Drawing for the job (mm, zero at the part's lowest x, y, z). A direction names the side the tool comes from. Coordinates: 2 decimals unless noted, no trailing zeros. Write each loop counter-clockwise with the first axis right and the second up, starting at its lowest first coordinate (ties: lowest second). Pieces come first, ordered by that corner, then holes. Notation, with made-up numbers: (11.25, -4.5) - (35.25, -4.5) arc R31 cw to (35.25, 31.5) - close; hole circle Ø2 at (42, -4). An arc over 180 degrees is marked (long way). Write each question's results on one line, items separated by ' | '.
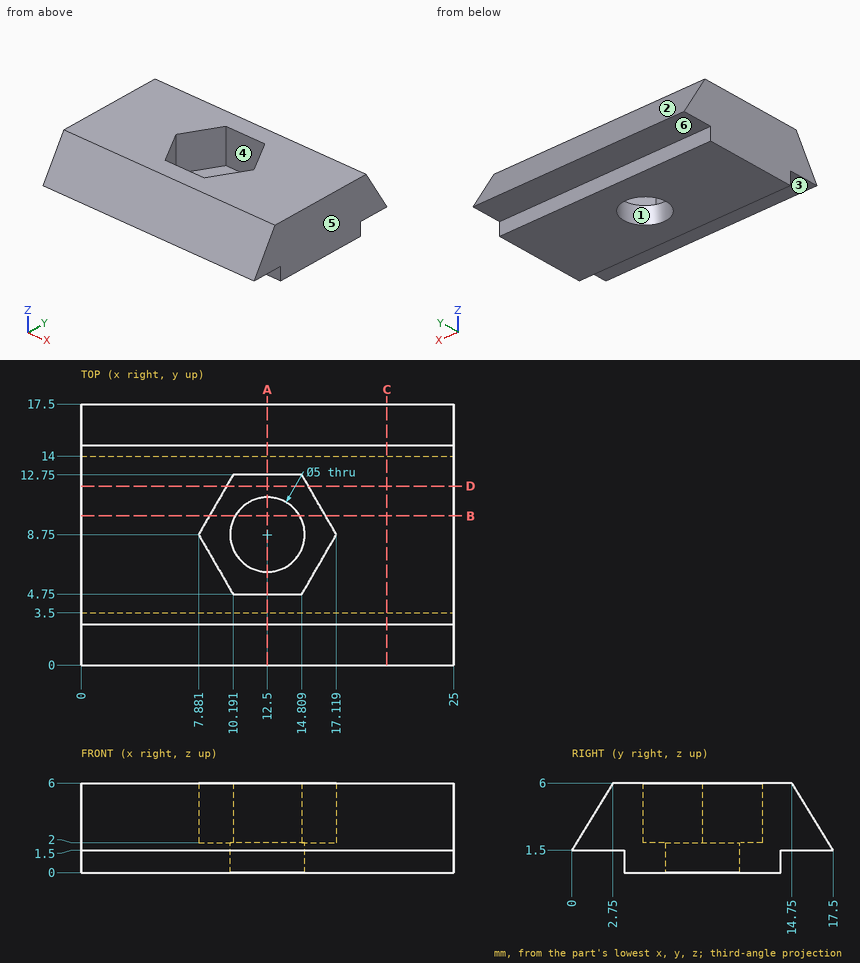
(1) Wall check: line 1 (X direction, y = 8.75, z = 0.8); line 2 (Z direction, x = 21.25, y = 14.5); line 3 (Y direction, x = 16, z = 0.75). Give the ranges that are in metal, low to high. Write a range as from..to.
Return value:
line 1: x = 0..10, 15..25 | line 2: z = 1.5..6 | line 3: y = 3.5..14
(2) Saw through at A-A on x = 12.5. Write the cut outline in (y, z).
Return value:
outline: (0, 1.5) - (3.5, 1.5) - (3.5, 0) - (6.25, 0) - (6.25, 2) - (4.75, 2) - (4.75, 6) - (2.75, 6) - close; (11.25, 0) - (14, 0) - (14, 1.5) - (17.5, 1.5) - (14.75, 6) - (12.75, 6) - (12.75, 2) - (11.25, 2) - close
(3) Saw through at C-C on x = 20.5. Write the cut outline in (y, z).
Return value:
outline: (0, 1.5) - (3.5, 1.5) - (3.5, 0) - (14, 0) - (14, 1.5) - (17.5, 1.5) - (14.75, 6) - (2.75, 6) - close
(4) Saw through at D-D on y = 12. Write the cut outline in (x, z), then the cut area to 3 significant figures.
Return value:
outline: (0, 0) - (25, 0) - (25, 6) - (15.24, 6) - (15.24, 2) - (9.76, 2) - (9.76, 6) - (0, 6) - close | area: 128 mm^2
(5) Flat gauge pins, fed straight in: P1, Ø3, axis at x = 8.5, y = 9.5, coming from the +Z side; P2, Ø2, axis at x = 12, z = 4.5, coming from the +Y side; P3, Ø1.2, axis at x = 12, z = 4.5, coming from the -Y side; P4, Ø1.6, axis at x = 9, z = 0.5, coming from the -Y side. Where does each tip first touch, or does it go through?
Return value:
P1: stops at z = 6 | P2: stops at y = 16.28 | P3: stops at y = 1.47 | P4: stops at y = 3.5
(6) 3-axis set-ups, long thin cutter, end or side, ignore diameter. For the marked faces 4, 5 and 6: which of +Z, -Z, +X, -X, +Y, -Y reach the whole face in a straight line?
Return value:
face 4: +Z | face 5: +Z, -Z, +X, +Y, -Y | face 6: -Z, +X, -X, +Y
(7) Two-plate mould, pull along Y, no slides. Class the marked faces 1, 2 and 3: released by +Y, released by -Y, zero draft, split by the parting line, or undercut.
Return value:
face 1: undercut | face 2: released by +Y | face 3: zero draft
(8) Saw through at B-B on y = 10. Write the cut outline in (x, z) (1 decimal).
Return value:
outline: (0, 0) - (10.3, 0) - (10.3, 2) - (8.6, 2) - (8.6, 6) - (0, 6) - close; (14.7, 0) - (25, 0) - (25, 6) - (16.4, 6) - (16.4, 2) - (14.7, 2) - close
